Part print with two shaded views. Sizes in mm from the minimum x, y, z corner. A direction names the side the tool comes from. Give positions to 0.01 mm unless a question says otherwise; leave off trailing zeros. Order: outer loops, then holes, each group sorted by start corner. A loop starts at its lowest first (then second) coordinate and runs counter-clockwise, first axis right, second up. Notation, with made-up numbers: (85, -31) -> (89, -31) arc R8 ccw to (89, -18) -> close; hole circle Ø6 at (-8.5, 76). An arc over 180 degrees is marked (long way). Answer as CSV lines item,"result".
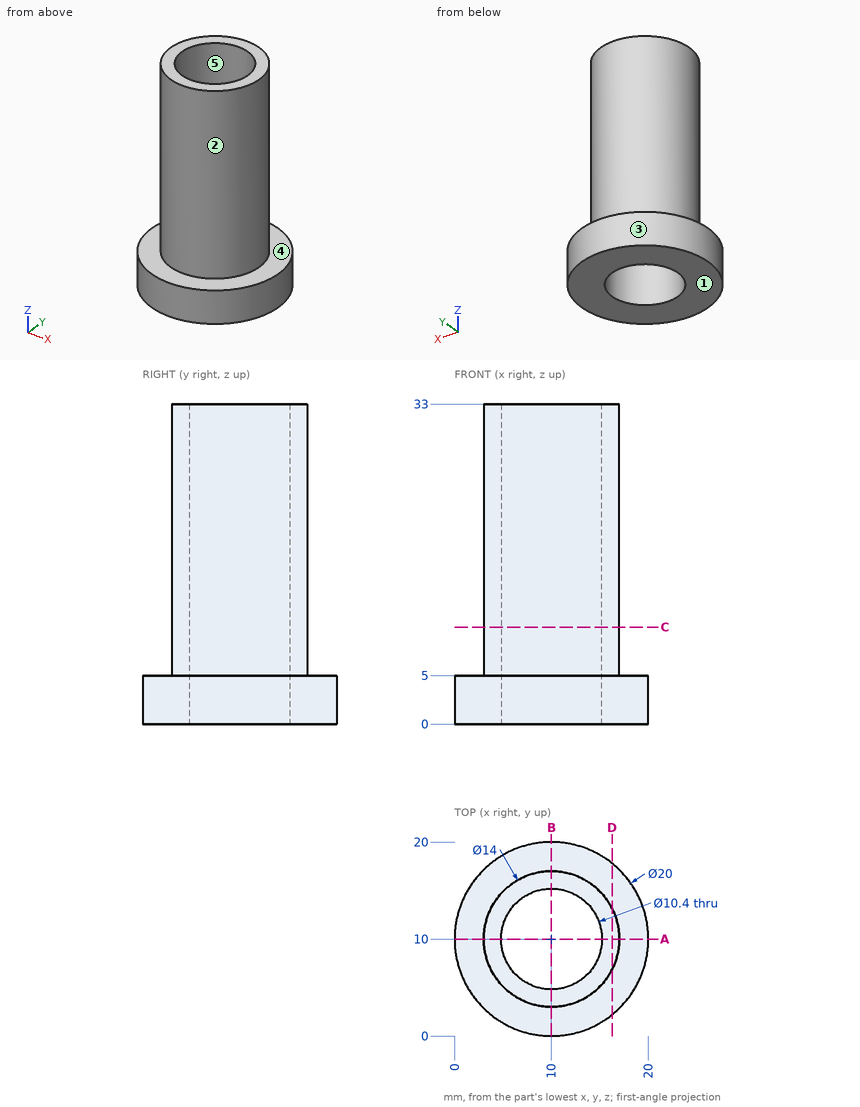
1) Band-saw the part on C-C, the plane z = 10. Write the cut outline in (x, y).
Data:
outline,"circle Ø14 at (10, 10); hole circle Ø10.4 at (10, 10)"
2) Which spindle directions (+Z, -Z, +X, -X, +Y, -Y) get a long thin tool onto all of the face, cutting with end or side? Do the marked faces 1 and 2. Say none if no direction does.
Data:
face 1,"-Z, +X, -X, +Y, -Y"
face 2,"+Z"
3) Band-saw the part on D-D, the plane x = 16.25. Write the cut outline in (y, z), then the cut area to 3 significant figures.
Data:
outline,"(2.19, 0) -> (17.81, 0) -> (17.81, 5) -> (13.15, 5) -> (13.15, 33) -> (6.85, 33) -> (6.85, 5) -> (2.19, 5) -> close"
area,"255 mm2"
4) Band-saw the part on A-A, the plane y = 10. Write the cut outline in (x, z), then the cut area to 3 significant figures.
Data:
outline,"(0, 0) -> (4.8, 0) -> (4.8, 33) -> (3, 33) -> (3, 5) -> (0, 5) -> close; (15.2, 0) -> (20, 0) -> (20, 5) -> (17, 5) -> (17, 33) -> (15.2, 33) -> close"
area,"149 mm2"
5) Wall check: line 1 along Y through (x, z) = (10, 15.5); line 2 along X through (y, z) = (14.5, 19.5). Give the ranges that are in metal, low to high. Write a range as [from, to].
Data:
line 1,"y = [3, 4.8], [15.2, 17]"
line 2,"x = [4.64, 7.39], [12.61, 15.36]"
6) Pull direction X, two halves, no side cores. Call the marked faces 3, 4 and 5: pulls with the +X half, pulls with the -X half, needs draft (parallel to the pull), parting line crosses it, or undercut.
Data:
face 3,"parting line crosses it"
face 4,"needs draft"
face 5,"undercut"
7) Pin check, flat tips, straight feed: P1, Ø3, axis at x = 9.5, y = 13, coming from the +Z side; P2, Ø4, axis at x = 12.5, y = 14, coming from the -Z side; P3, Ø10, axis at x = 11.5, z = 13, coming from the -Y side; P4, Ø2, axis at y = 12.5, z = 28.5, coming from the -X side. Stop position of each tip, or through.
Data:
P1,"passes through"
P2,"stops at z = 0"
P3,"stops at y = 3"
P4,"stops at x = 3.16"
